Input: part model. Units: mm. Frame: model coordinates. Face numbers are marked on the shaded views. A direction names the side the tool comes from. Coordinates: 2 decimals unless noted, no trailing zeros. Write each loop counter-clockwise with the first axis right and the second up, starting at its lowest first coordinate (ties: lowest second). Pieces come first, ordered by that corner, then holes. Notation, with made-up numbers: M 40,-22.5 L 62,-22.5 A35 ccw 62,9.5 Z; hole C -26.75,58.25 d2. An arc over 180 degrees is marked long. Use CSV: the item, a comma, the result in double quotes.
Autodesk Inventor part; units mm, degrees
ref_plane "YZ Plane" through (0, 0, 0) normal (1, 0, 0) x (0, 1, 0)
ref_plane "XZ Plane" through (0, 0, 0) normal (0, 1, 0) x (-1, 0, 0)
ref_plane "XY Plane" through (0, 0, 0) normal (0, 0, 1) x (1, 0, 0)
sketch "Sketch1" plane through (0, 0, 0) normal (0, 0, 1) x (1, 0, 0)
  line L0 (0, 0) -> (44.45, 0)
  line L1 (44.45, 0) -> (44.45, 12.7)
  line L2 (44.45, 12.7) -> (12.7, 12.7)
  line L3 (12.7, 12.7) -> (12.7, 31.75)
  line L4 (12.7, 31.75) -> (0, 31.75)
  line L5 (0, 31.75) -> (0, 0)
  dimension "d0" = 44.45
  dimension "d1" = 12.7
  dimension "d2" = 31.75
  dimension "d3" = 19.05
extrude "Extrusion1" add sketch "Sketch1" along normal blind 31.75
sketch "Sketch2" plane through (0, 31.75, 0) normal (0, 1, 0) x (1, 0, 0)
  line L0 (0, -31.8326) -> (0, -25.4826) construction
  line L1 (0, 0) -> (0, -31.75) construction
  line L2 (0, -25.4826) -> (12.7, -25.4826)
  line L3 (12.7, 0) -> (12.7, -31.75)
  line L4 (12.7, -25.4826) -> (12.7, -6.4326)
  line L5 (12.7, -6.4326) -> (0, -6.4326)
  line L6 (0, -6.4326) -> (0, -25.4826)
  dimension "d6" = 6.35
  dimension "d7" = 19.05
extrude "Extrusion2" cut sketch "Sketch2" against normal blind 6.35
sketch "Sketch4" plane through (12.7, 12.7, 0) normal (0, 1, 0) x (1, 0, 0)
  line L0 (31.75, 0) -> (31.75, -31.75) construction
  line L1 (31.75, -31.75) -> (31.75, -19.05) construction
  line L2 (31.75, -19.05) -> (12.7, -19.05)
  line L3 (12.7, -19.05) -> (12.7, -12.7)
  line L4 (12.7, -12.7) -> (31.75, -12.7)
  line L5 (31.75, -12.7) -> (31.75, -19.05)
  point P0 (-12.7, 0)
  dimension "d10" = 12.7
  dimension "d11" = 19.05
  dimension "d12" = 6.35
extrude "Extrusion3" cut sketch "Sketch4" against normal blind 19.05
properties part number "Aluminum Part" material "Aluminum 6061"
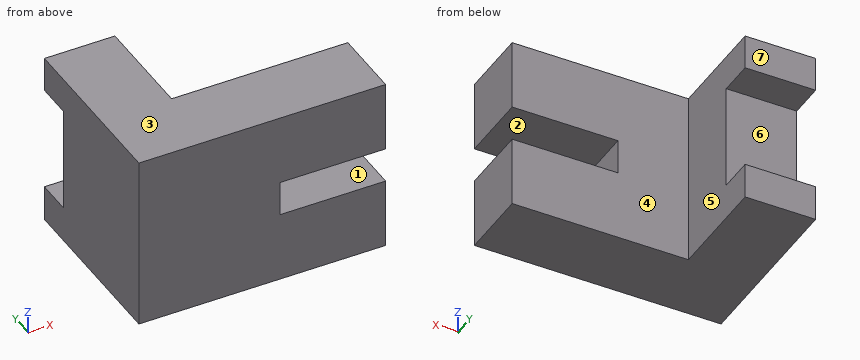
1. Access query for the marked faces 5, 6 and 7. Directions: +Z, -Z, +X, -X, +Y, -Y. A direction counts if a zero-diameter tool reaches every point of the face in a straight line with its end or side. Return the directions, or none.
Resolved:
face 5,"+Z, -Z, +X, +Y"
face 6,"+X, -X, +Y"
face 7,"+Z, -Z, +X, -X, +Y"
2. Section A-A (x = 41). Return loops of the section in (y, z).
Resolved:
outline,"M 0,0 L 12.7,0 L 12.7,12.7 L 0,12.7 Z; M 0,19.05 L 12.7,19.05 L 12.7,31.75 L 0,31.75 Z"
3. Section B-B (x = 8). Return loops of the section in (y, z).
Resolved:
outline,"M 0,0 L 31.75,0 L 31.75,6.43 L 25.4,6.43 L 25.4,25.48 L 31.75,25.48 L 31.75,31.75 L 0,31.75 Z"
4. Mould query, pull axis Z, two halves, no side actions, for the marked faces 1, 2, 3 and 4. Classes: pulls with the +Z half, pulls with the -Z half, needs draft (parallel to the pull), parting line crosses it, or undercut.
Resolved:
face 1,"undercut"
face 2,"undercut"
face 3,"pulls with the +Z half"
face 4,"needs draft"
5. Section C-C (y = 12). Return loops of the section in (x, z).
Resolved:
outline,"M 0,0 L 44.45,0 L 44.45,12.7 L 25.4,12.7 L 25.4,19.05 L 44.45,19.05 L 44.45,31.75 L 0,31.75 Z"
6. Section D-D (z = 23.5). Return loops of the section in (x, y).
Resolved:
outline,"M 0,0 L 44.45,0 L 44.45,12.7 L 12.7,12.7 L 12.7,25.4 L 0,25.4 Z"
7. Contact query for flat-ended pins moving along their axis: pin 1 Ø7 at (y, z) = (6, 16.5) entering from +X; pin 2 Ø6 at (x, z) = (40, 4) entering from +Y; pin 3 Ø4 at (x, z) = (7.5, 18.5) entering from +Y; pin 4 Ø5.5 at (y, z) = (23.5, 23) entering from +X. Output: stop coordinate, or through.
Resolved:
pin 1,"stops at x = 44.45"
pin 2,"stops at y = 12.7"
pin 3,"stops at y = 25.4"
pin 4,"stops at x = 12.7"
8. Material intervals for line 1 (Z direction, x = 32, y = 3.5); line 2 (Z direction, x = 9.5, y = 28); line 3 (X direction, y = 21, z = 13.5), sorted ascending. Write a range as [from, to].
Resolved:
line 1,"z = [0, 12.7], [19.05, 31.75]"
line 2,"z = [0, 6.43], [25.48, 31.75]"
line 3,"x = [0, 12.7]"
